```python
from build123d import *

# Parameters (mm, degrees)
F0_R     = 38.1
F1_DEPTH = 19.05
F2_SIZE  = 6.35
F3_R     = 25.4
F4_DEPTH = 12.7
F5_SIZE  = 6.35


with BuildPart() as f1:
    # F0 (on Top) → F1 (new body)
    with BuildSketch(Plane.XY):
        Circle(F0_R)
    extrude(amount=F1_DEPTH)

    # F2
    f2_edges = [f1.edges().sort_by_distance(p)[0] for p in [
        (-38.1, 0, 19.05),
    ]]
    chamfer(f2_edges, length=F2_SIZE)

    # F3 (on face) → F4 (cut)
    with BuildSketch(Plane(origin=(0, 0, 0), x_dir=(1, 0, 0), z_dir=(0, 0, -1))):
        Circle(F3_R)
    extrude(amount=-F4_DEPTH, mode=Mode.SUBTRACT)

    # F5
    f5_edges = [f1.edges().sort_by_distance(p)[0] for p in [
        (-25.4, 0, 12.7),
    ]]
    chamfer(f5_edges, length=F5_SIZE)


solid = f1.part
```
Part model, mm, in its own coordinate system. A direction names the side the tool comes from. Coordinates: 2 decimals unless noted, no trailing zeros. Write each loop counter-clockwise with the first axis right and the second up, starting at its lowest first coordinate (ties: lowest second). Pieces come first, ordered by that corner, then holes.
Item 1: Slice it at B-B (z = 8.25). Write the cut outline in (x, y).
Item 2: Pin check, flat tips, straight feed: pin 1 (6 mm diameter, centred on y = -6, z = 9, fed in from -X); pin 2 (3 mm diameter, centred on x = 27, z = 3, fed in from +Y); pin 3 (8 mm diameter, centred on x = 22, z = 4, fed in from +Y); pin 4 (8 mm diameter, centred on x = -22.5, y = 23.5, fed in from -Z). Stop position of each tip, or through.
Item 3: Mould opens along Y. For faces 1 (the face through (-30.235, -23.183, 6.261)), 2 (the face through (-5.506, 24.796, 3.131)), 3 (the face through (8, -25, 0)) say: released by +Y, released by -Y, zero draft, split by the parting line, or undercut.
Item 4: Slice it at D-D (z = 15.25). Write the cut outline in (x, y).
Item 5: Probe line 1 (Y direction, x = 0, z = 3.5); line 2 (Y direction, x = 6.5, z = 5); line 3 (X direction, y = -10.5, z = 10). List the from-to ranges inside material, lowest first.
Item 6: Slice it at A-A (x = 0). Write the cut outline in (y, z).
Item 7: Which spindle directions (+Z, -Z, +X, -X, +Y, -Y) get a long thin tool onto all of the face, cutting with end or side? Do faces 4 (the face through (-25.44, -19.51, 18.74)), 5 (the face through (0, 0, 12.7)). Say none if no direction does.
Results found:
1. outline: circle Ø76.2 at (0, 0); hole circle Ø47 at (0, 0)
2. pin 1: stops at x = -37.98
2. pin 2: stops at y = 28.31
2. pin 3: stops at y = 33.58
2. pin 4: stops at z = 0
3. face 1: split by the parting line
3. face 2: undercut
3. face 3: zero draft
4. outline: circle Ø71.1 at (0, 0)
5. line 1: y = -38.1 to -25.4, 25.4 to 38.1
5. line 2: y = -37.54 to -24.55, 24.55 to 37.54
5. line 3: x = -36.62 to -19.05, 19.05 to 36.62
6. outline: (-38.1, 0) - (-25.4, 0) - (-25.4, 6.35) - (-19.05, 12.7) - (19.05, 12.7) - (25.4, 6.35) - (25.4, 0) - (38.1, 0) - (38.1, 12.7) - (31.75, 19.05) - (-31.75, 19.05) - (-38.1, 12.7) - close
7. face 4: +Z
7. face 5: -Z
